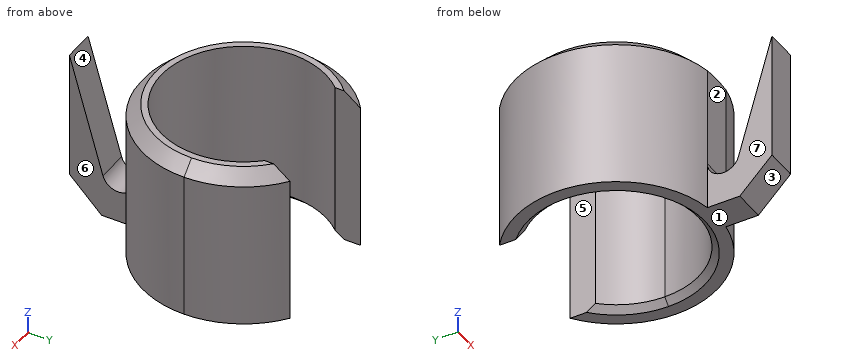
```python
from build123d import *

# Parameters (mm, degrees)
F1_DEPTH = 25.4
F3_DEPTH = 25.4
F5_DEPTH = 25.4
F6_SIZE  = 5.08
F7_SIZE  = 1
F8_SIZE  = 2


with BuildPart() as f1:
    # F0 (on Top) → F1 (new body)
    with BuildSketch(Plane.XY):
        with BuildLine():
            Line((9.5, 12.8743931896), (9.5, 8.8741196746))
            ThreePointArc((9.5, 8.8741196746), (12.0933866224, 4.7696960071), (13, 0))
            ThreePointArc((13, 0), (-4.7696960071, -12.0933866224), (-9.5, 8.8741196746))
            Line((-9.5, 8.8741196747), (-9.5, 12.8743931896))
            ThreePointArc((-9.5, 12.8743931896), (-7.2111025509, -14.2828568571), (16, 0))
            ThreePointArc((16, 0), (14.2828568571, 7.2111025509), (9.5, 12.8743931896))
        make_face()
    extrude(amount=F1_DEPTH)

    # F2 (on face) → F3 (join, through all)
    with BuildSketch(Plane(origin=(0, 0, 0), x_dir=(1, 0, 0), z_dir=(0, 0, -1))):
        with BuildLine():
            Line((2.5, 15.8034806293), (2.5, 26))
            Line((2.5, 26), (-2.5, 26))
            Line((-2.5, 26), (-2.5, 15.8034806293))
            ThreePointArc((-2.5, 15.8034806293), (0, 16), (2.5, 15.8034806293))
        make_face()
    extrude(amount=-F3_DEPTH)

    # F4 (on face) → F5 (cut)
    with BuildSketch(Plane(origin=(-2.5, 0, 0), x_dir=(0, -1, 0), z_dir=(-1, 0, 0))):
        with BuildLine():
            ThreePointArc((20.8034806293, 7.5), (20.7794696728, 7.1543437309), (20.7078980242, 6.8153270919))
            Line((20.7078980242, 6.8153270919), (26, 25.4000000001))
            Line((26, 25.4), (15.8034806293, 25.4))
            Line((15.8034806293, 25.4), (15.8034806293, 7.4999999981))
            ThreePointArc((15.8034806293, 7.4999999981), (18.3034806283, 10), (20.8034806293, 7.5))
        make_face()
        with BuildLine():
            ThreePointArc((15.8034806293, 7.4999999981), (17.9578243611, 5.0240109563), (20.7078980242, 6.8153270919))
            ThreePointArc((20.7078980242, 6.8153270919), (20.7794696728, 7.1543437309), (20.8034806293, 7.5))
            ThreePointArc((20.8034806293, 7.5), (18.3034806283, 10), (15.8034806293, 7.4999999981))
        make_face()
    extrude(amount=-F5_DEPTH, mode=Mode.SUBTRACT)

    # F6
    f6_edges = [f1.edges().sort_by_distance(p)[0] for p in [
        (0, -26, 0),
    ]]
    chamfer(f6_edges, length=F6_SIZE)

    # F7
    f7_edges = [f1.edges().sort_by_distance(p)[0] for p in [
        (0, -13, 0),
    ]]
    chamfer(f7_edges, length=F7_SIZE)

    # F8
    f8_edges = [f1.edges().sort_by_distance(p)[0] for p in [
        (14.282857, 7.211103, 25.4),
    ]]
    chamfer(f8_edges, length=F8_SIZE)


solid = f1.part
```
Could you check a few things on this model? Use its own coordinates, in mm. Face numbers are marked on the shaded views. A direction names the side the tool comes from. Coordinates: 2 decimals unless noted, no trailing zeros. Order: outer loops, then holes, each group sorted by start corner. A loop starts at its lowest first (then second) coordinate and runs counter-clockwise, first axis right, second up. Notation, with made-up numbers: M -24,7.25 L 4,7.25 A13 ccw 4,25.25 Z; hole C 85.5,50.5 d1. An arc over 180 degrees is marked long. Use one line per item in the form item = value. Start each with the question number.
1. We'd pull the mould along Y, two halves only. Please class the marked faces 1, 2 and 3: +Y half, -Y half, draft (parallel to the pull), parting line (faces both ways), or undercut.
2. Suppose I cut it at A-A on z = 17. Write out the boundary of the cut face in (x, y).
3. Suppose I cut it at B-B on x = 0. Write out the boundary of the cut face in (y, z), then the cut area to 3 significant figures.
4. Please list where these lines run through material, in increasing order: line 1 (X direction, y = -2, z = 19.25); line 2 (X direction, y = -12, z = 22.5); line 3 (X direction, y = -23.5, z = 3).
5. Suppose I cut it at D-D on z = 20.5. Write out the boundary of the cut face in (x, y).
6. For pin 1 (1.5 mm diameter, centred on x = -4.5, z = 9.5, fed in from -Y); pin 2 (2 mm diameter, centred on x = -6, z = 19, fed in from +Y); pin 3 (3 mm diameter, centred on y = 11.5, z = 7, fed in from -X); pin 4 (8 mm diameter, centred on x = -3.5, y = -7.5, fed in from -Z), each with a flat end and sliding along its axis, tell me the tip position at first contact or that it passes through.
7. Suppose I cut it at C-C on z = 3.25. Write out the boundary of the cut face in (x, y).
8. On a 3-axis mill with a long thin cutter (end or side, diameter ignored), from which of +Z, -Z, +X, -X, +Y, -Y can I reach the whole of each face in a straight line? I mean the marked faces 4, 5, 6 and 7. Say none if no direction works.
Geometry says:
q1.face_1 = draft
q1.face_2 = undercut
q1.face_3 = -Y half
q2.outline = M -9.5,8.87 L -9.5,12.87 A16 ccw -2.5,-15.8 L 2.5,-15.8 A16 ccw 9.5,12.87 L 9.5,8.87 A13 cw long Z; M -2.5,-26 L 2.5,-26 L 2.5,-23.61 L -2.5,-23.61 Z
q3.outline = M -26,5.08 L -20.92,0 L -14,0 L -13,1 L -13,25.4 L -14,25.4 L -15.8,23.6 L -15.8,7.5 A2.5 cw -20.71,6.82 L -26,25.4 Z
q3.area = 168 mm^2
q4.line_1 = -15.87 to -12.85, 12.85 to 15.87
q4.line_2 = -10.58 to -5, 5 to 10.58
q4.line_3 = -2.5 to 2.5
q5.outline = M -9.5,8.87 L -9.5,12.87 A16 ccw -2.5,-15.8 L 2.5,-15.8 A16 ccw 9.5,12.87 L 9.5,8.87 A13 cw long Z; M -2.5,-26 L 2.5,-26 L 2.5,-24.6 L -2.5,-24.6 Z
q6.pin_1 = -15.55
q6.pin_2 = -10.95
q6.pin_3 = -12.49
q6.pin_4 = through
q7.outline = M -9.5,8.87 L -9.5,12.87 A16 ccw -2.5,-15.8 L -2.5,-24.17 L 2.5,-24.17 L 2.5,-15.8 A16 ccw 9.5,12.87 L 9.5,8.87 A13 cw long Z
q8.face_4 = +Z, +X, -X
q8.face_5 = +Z, -Z, +Y
q8.face_6 = +Z, -Z, +X, -Y
q8.face_7 = +Z, -Z, -X, -Y
